Geometry: final body of the model. Coordinates: model frame, mm. A direction names the side the tool comes from. Coordinates: 2 decimals unless noted, no trailing zeros. Order: outer loops, then holes, each group sorted by start corner. A loop starts at its lowest first (then second) coordinate and runs counter-clockwise, first axis right, second up. Notation, with made-up numbers: M 30.5,62 L 45.5,62 A30 cw 45.5,88 Z; hole C 70.25,6.25 d10. An arc over 180 degrees is marked long. Write item = value, one per line.
from build123d import *

# Parameters (mm, degrees)
F0_W     = 8.001
F0_H     = 8
F1_DEPTH = 9.6
F2_R     = 2.425
F3_DEPTH = 1.7
F4_T     = -1.5


with BuildPart() as f1:
    # F0 (on Top) → F1 (new body)
    with BuildSketch(Plane.XY):
        Rectangle(F0_W, F0_H)
    extrude(amount=F1_DEPTH)

    # F2 (on face) → F3 (join)
    with BuildSketch(Plane.XY.offset(9.6)):
        Circle(F2_R)
    extrude(amount=F3_DEPTH)

    # F4
    f4_openings = [f1.faces().sort_by_distance(p)[0] for p in [
        (0, 0, 0),
    ]]
    offset(amount=F4_T, openings=f4_openings, kind=Kind.INTERSECTION)


solid = f1.part
1) Section D-D, the plane z = 3.5. Return loops of the section in (x, y).
Numbers:
outline = M -4,-4 L 4,-4 L 4,4 L -4,4 Z; hole M -2.5,-2.5 L 2.5,-2.5 L 2.5,2.5 L -2.5,2.5 Z
2) Pin query (flat end, axial travel): pin 1 (2.5 mm diameter, centred on x = 0, y = -0.5, fed in from -Z); pin 2 (1 mm diameter, centred on x = 3, y = -2, fed in from +Z). Return the tip coordinate at first contact, or that it passes through.
Numbers:
pin_1 = 8.1
pin_2 = 9.6
3) Section B-B, the plane x = 0. Return loops of the section in (y, z) (3 decimals).
Numbers:
outline = M -4,0 L -2.5,0 L -2.5,8.1 L -0.925,8.1 L -0.925,9.8 L 0.925,9.8 L 0.925,8.1 L 2.5,8.1 L 2.5,0 L 4,0 L 4,9.6 L 2.425,9.6 L 2.425,11.3 L -2.425,11.3 L -2.425,9.6 L -4,9.6 Z
4) Mould query, pull axis X, two halves, no side actions, for faces 1 (the face through (4, 0, 5)), 2 (the face through (0, 0, 11.3)), 3 (the face through (2.5, 0, 4)). Classes: pulls with the +X half, pulls with the -X half, needs draft (parallel to the pull), parting line crosses it, or undercut.
Numbers:
face_1 = pulls with the +X half
face_2 = needs draft
face_3 = undercut
5) Line query: L1, parallel to X at y = 0, z = 8.9 (1 decimal); L2, parallel to Y at x = 0, z = 8.65 (3 decimals); L3, parallel to X at y = -0.75, z = 7.75. Output: solid intervals per line, ascending.
Numbers:
L1 = -4 to -0.9, 0.9 to 4
L2 = -4 to -0.925, 0.925 to 4
L3 = -4 to -2.5, 2.5 to 4
6) Section C-C, the plane y = 0. Return loops of the section in (x, z) (1 decimal).
Numbers:
outline = M -4,0 L -2.5,0 L -2.5,8.1 L -0.9,8.1 L -0.9,9.8 L 0.9,9.8 L 0.9,8.1 L 2.5,8.1 L 2.5,0 L 4,0 L 4,9.6 L 2.4,9.6 L 2.4,11.3 L -2.4,11.3 L -2.4,9.6 L -4,9.6 Z
7) Set-up query: faces 4 (the face through (0, -4, 5)), 5 (the face through (0, 2.5, 4)), 6 (the face through (2, 2, 9.6)). Return all of +Z, -Z, +X, -X, +Y, -Y with unobstructed straight access to the full face (end or side cutting, diameter ignored); none if empty.
Numbers:
face_4 = +Z, -Z, +X, -X, -Y
face_5 = -Z
face_6 = +Z
